```python
from build123d import *

# Parameters (mm, degrees)
F0_W     = 10
F0_H     = 75
F1_DEPTH = 25


with BuildPart() as f1:
    # F0 (on Front) → F1 (new body)
    with BuildSketch(Plane.XZ):
        Polygon((10, 162.5), (-10, 162.5), (-10, -162.5), (10, -162.5), (10, -137.5), (10, -62.5), (10, 62.5), (10, 137.5), align=None)
        Polygon((30, 162.5), (10, 162.5), (10, 137.5), (20, 137.5), (30, 137.5), align=None)
        with Locations((15, 100)):
            Rectangle(F0_W, F0_H)
        Polygon((10, -137.5), (10, -162.5), (30, -162.5), (30, -137.5), (20, -137.5), align=None)
        with Locations((15, -100)):
            Rectangle(F0_W, F0_H)
    extrude(amount=F1_DEPTH)


solid = f1.part
```
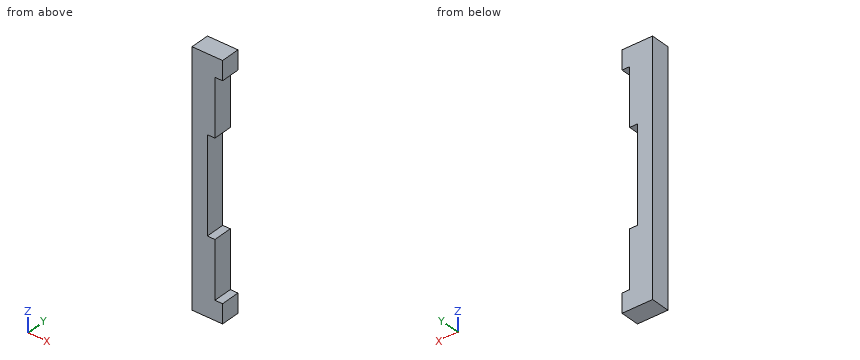
Geometry: final body of the model. Coordinates: model frame, mm. Round coordinates to 2 decimals unless told otherwise and drop trailing zeros. Order: outer loops, then holes, each group sorted by start corner. A loop starts at its lowest first (then second) coordinate and runs counter-clockwise, first axis right, second up. Notation, with made-up numbers: M -3.75,73 L 50.25,73 A25 ccw 50.25,86 Z; hole C -20,13.25 d5. An arc over 180 degrees is marked long. One line per item, written item: value.
(1) Cut plane D-D (z = 122.5). Return the cut outline in (x, y), and give its area (3 significant figures).
Result sheet:
outline: M -10,-25 L 20,-25 L 20,0 L -10,0 Z
area: 750 mm2
(2) Line query: probe 1 along Z at (x, y) = (16.5, -4.75); probe 2 along Z at (x, y) = (27, -9.5); probe 3 along X at (y, z) = (-15.5, -66). Output: solid intervals per line, ascending. Write a range as [from, to].
Result sheet:
probe 1: [-162.5, -62.5], [62.5, 162.5]
probe 2: [-162.5, -137.5], [137.5, 162.5]
probe 3: [-10, 20]
(3) Pin query (flat end, axial travel): P1, Ø7.5, axis at y = -18.5, z = 99.5, coming from the +X side; P2, Ø3, axis at y = -17.5, z = -58.5, coming from the +X side. Return the tip coordinate at first contact, or that it passes through.
Result sheet:
P1: x = 20
P2: x = 10
(4) Cut plane B-B (y = -17.75). Return the cut outline in (x, z), and give its area (3 significant figures).
Result sheet:
outline: M -10,-162.5 L 30,-162.5 L 30,-137.5 L 20,-137.5 L 20,-62.5 L 10,-62.5 L 10,62.5 L 20,62.5 L 20,137.5 L 30,137.5 L 30,162.5 L -10,162.5 Z
area: 9,000 mm2
(5) Cut plane C-C (z = -6.5). Return the cut outline in (x, y).
Result sheet:
outline: M -10,-25 L 10,-25 L 10,0 L -10,0 Z
(6) Cut plane A-A (x = 14). Return the cut outline in (y, z), and give its area (3 significant figures).
Result sheet:
outline: M -25,-162.5 L 0,-162.5 L 0,-62.5 L -25,-62.5 Z; M -25,62.5 L 0,62.5 L 0,162.5 L -25,162.5 Z
area: 5,000 mm2
